from build123d import *

# Parameters (mm, degrees)
F0_W     = 24
F0_H     = 30.8
F0_R     = 7.95
F1_DEPTH = 28.5
F3_W     = 15.4
F3_H     = 28.5
F4_DEPTH = 10
F2_W     = 15.4
F2_H     = 28.5
F5_DEPTH = 10
F6_R     = 1.6
F7_DEPTH = 30.801
F0_R_2   = 4.75
F8_DEPTH = 1.5
F9_R     = 3


with BuildPart() as f1:
    # F0 (on Top) → F1 (new body)
    with BuildSketch(Plane.XY):
        Rectangle(F0_W, F0_H)
        with Locations((0, 5.75)):
            Circle(F0_R, mode=Mode.SUBTRACT)
    extrude(amount=F1_DEPTH)

    # F3 (on face) → F4 (join)
    with BuildSketch(Plane.YZ.offset(12)):
        with Locations((-7.7, 14.25)):
            Rectangle(F3_W, F3_H)
    extrude(amount=F4_DEPTH)

    # F2 (on face) → F5 (join)
    with BuildSketch(Plane(origin=(-12, 0, 0), x_dir=(0, -1, 0), z_dir=(-1, 0, 0))):
        with Locations((7.7, 14.25)):
            Rectangle(F2_W, F2_H)
    extrude(amount=F5_DEPTH)

    # F6 (on face) → F7 (cut, through all)
    with BuildSketch(Plane(origin=(0, 15.4, 0), x_dir=(-1, 0, 0), z_dir=(0, 1, 0))):
        with Locations((-17, 14.25)):
            Circle(F6_R)
        with Locations((17, 14.25)):
            Circle(F6_R)
    extrude(amount=-F7_DEPTH, mode=Mode.SUBTRACT)

    # F0 (on Top) → F8 (join)
    with BuildSketch(Plane.XY):
        with Locations((0, 5.75)):
            Circle(F0_R)
        with Locations((0, 5.75)):
            Circle(F0_R_2, mode=Mode.SUBTRACT)
    extrude(amount=F8_DEPTH)

    # F9
    f9_edges = [f1.edges().sort_by_distance(p)[0] for p in [
        (12, 15.4, 14.25),
        (22, 0, 14.25),
        (-22, 0, 14.25),
        (-12, 15.4, 14.25),
    ]]
    fillet(f9_edges, radius=F9_R)


solid = f1.part
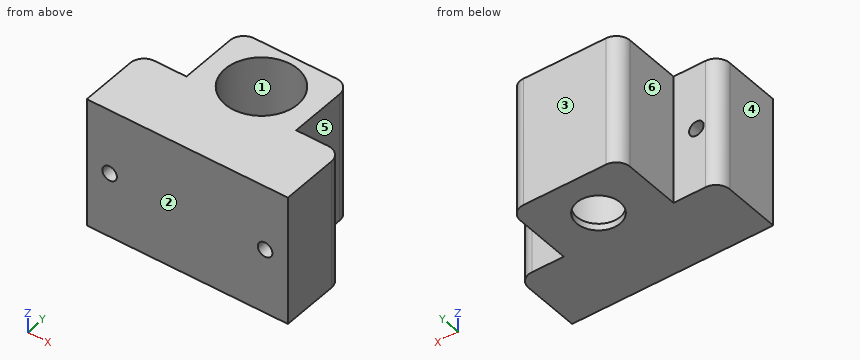
Part model, mm, in its own coordinate system. Face numbers are marked on the shaded views. A direction names the side the tool comes from. Give positions to 0.01 mm unless a question says otherwise; leave off trailing zeros. Write each loop counter-clockwise with the first axis right and the second up, starting at its lowest first coordinate (ties: lowest second). Pieces come first, ordered by that corner, then holes.
1) Two-plate mould, pull along Y, no slides. Class the marked faces 1, 2 and 3: released by +Y, released by -Y, zero draft, split by the parting line, or undercut.
Resolved:
face 1: undercut
face 2: released by -Y
face 3: released by +Y
2) Cut at C-C on x = 0. Write the cut outline in (y, z).
Resolved:
outline: (-15.4, 0) - (1, 0) - (1, 1.5) - (-2.2, 1.5) - (-2.2, 28.5) - (-15.4, 28.5) - close; (10.5, 0) - (15.4, 0) - (15.4, 28.5) - (13.7, 28.5) - (13.7, 1.5) - (10.5, 1.5) - close
3) Cut at D-D on z = 17.75. Write the cut outline in (x, y).
Resolved:
outline: (-22, -15.4) - (22, -15.4) - (22, -3) arc R3 ccw to (19, 0) - (12, 0) - (12, 12.4) arc R3 ccw to (9, 15.4) - (-9, 15.4) arc R3 ccw to (-12, 12.4) - (-12, 0) - (-19, 0) arc R3 ccw to (-22, -3) - close; hole circle Ø15.9 at (0, 5.75)
4) Probe L1, parallel to Z at x = -17, y = -7.75; L2, parallel to Y at x = 13, z = 3.75; L3, parallel to Y at x = -4.5, z = 1.75. List the from-to ranges inside material, lowest first.
Resolved:
L1: z = 0 to 12.65, 15.85 to 28.5
L2: y = -15.4 to 0
L3: y = -15.4 to -0.8, 12.3 to 15.4
5) Cut at B-B on y = 5.75. Write the cut outline in (x, z).
Resolved:
outline: (-12, 0) - (-4.75, 0) - (-4.75, 1.5) - (-7.95, 1.5) - (-7.95, 28.5) - (-12, 28.5) - close; (4.75, 0) - (12, 0) - (12, 28.5) - (7.95, 28.5) - (7.95, 1.5) - (4.75, 1.5) - close
6) Which spindle directions (+Z, -Z, +X, -X, +Y, -Y) get a long thin tool onto all of the face, cutting with end or side? Do the marked faces 4, 5 and 6. Say none if no direction does.
Resolved:
face 4: +Z, -Z, -X, +Y, -Y
face 5: +Z, -Z, +X, +Y
face 6: +Z, -Z, -X, +Y
7) Pin check, flat tips, straight feed: pin 1 (5 mm diameter, centred on x = 0, y = 9.5, fed in from +Z); pin 2 (10 mm diameter, centred on y = 2.5, z = 16.5, fed in from -X); pin 3 (5.5 mm diameter, centred on x = 17, z = 21, fed in from +Y); pin 4 (2.5 mm diameter, centred on x = 17, z = 14.25, fed in from +Y). Stop position of each tip, or through.
Resolved:
pin 1: stops at z = 1.5
pin 2: stops at x = -21.96
pin 3: stops at y = 0
pin 4: passes through
8) Cut at A-A on z = 14.25. Write the cut outline in (x, y), then the cut area to 3 significant figures.
Resolved:
outline: (-22, -15.4) - (-18.6, -15.4) - (-18.6, 0) - (-19, 0) arc R3 ccw to (-22, -3) - close; (-15.4, -15.4) - (15.4, -15.4) - (15.4, 0) - (12, 0) - (12, 12.4) arc R3 ccw to (9, 15.4) - (-9, 15.4) arc R3 ccw to (-12, 12.4) - (-12, 0) - (-15.4, 0) - close; (18.6, -15.4) - (22, -15.4) - (22, -3) arc R3 ccw to (19, 0) - (18.6, 0) - close; hole circle Ø15.9 at (0, 5.75)
area: 742 mm2
